```python
from build123d import *

# Parameters (mm, degrees)
BOSS_EXTRUDE1_DEPTH  = 15
BOSS_EXTRUDE8_DEPTH  = 10
SKETCH5_W            = 15
SKETCH5_H            = 15
BOSS_EXTRUDE10_DEPTH = 10
CUT_EXTRUDE4_DEPTH   = 10
BOSS_EXTRUDE11_DEPTH = 10


with BuildPart() as part:
    # Sketch1 → Boss-Extrude1 (new body)
    with BuildSketch(Plane.XY):
        Polygon((-20, -5), (-20, 5), (-10, 5), (-10, 10), (0, 10), (0, 0), (-10, 0), (-10, -5), align=None)
    extrude(amount=BOSS_EXTRUDE1_DEPTH)

    # Sketch2 → Boss-Extrude8 (add)
    with BuildSketch(Plane(origin=(-10, 0, 0), x_dir=(0, 0, -1), z_dir=(1, 0, 0))):
        Polygon((0, 0), (0, -5), (-15, 0), align=None)
    extrude(amount=BOSS_EXTRUDE8_DEPTH)

    # Sketch5 → Boss-Extrude10 (add)
    with BuildSketch(Plane(origin=(0, 0, 0), x_dir=(0, 0, -1), z_dir=(1, 0, 0))):
        with Locations((-7.5, 2.5)):
            Rectangle(SKETCH5_W, SKETCH5_H)
    extrude(amount=BOSS_EXTRUDE10_DEPTH)

    # Sketch6 → Cut-Extrude4 (cut)
    with BuildSketch(Plane(origin=(10, 0, 0), x_dir=(0, 0, -1), z_dir=(1, 0, 0))):
        Polygon((-15, -5), (0, 0), (0, -5), align=None)
    extrude(amount=-CUT_EXTRUDE4_DEPTH, mode=Mode.SUBTRACT)

    # Sketch7 → Boss-Extrude11 (add)
    with BuildSketch(Plane.ZY.offset(10)):
        Polygon((0, 5), (0, 15), (15, 5), align=None)
    extrude(amount=BOSS_EXTRUDE11_DEPTH)


solid = part.part
```
Model file for the job. Use its own axes, mm. A direction names the side the tool comes from. Give positions to 0.01 mm unless a question says otherwise; leave off trailing zeros. Write each loop counter-clockwise with the first axis right and the second up, starting at its lowest first coordinate (ties: lowest second). Pieces come first, ordered by that corner, then holes. Notation, with made-up numbers: (7, 33) -> (55, 33) arc R27 cw to (55, 58) -> close; hole circle Ø11 at (79, 16.25). An arc over 180 degrees is marked (long way). Use CSV: the item, a comma, the result in double quotes. Start each with the question number.
1) Two-plate mould, pull along X, no slides. Class faces 1 (the flat face through (-5.07, -2.535, 7.395)), 2 (the flat face through (0, 10, 8)), 3 (the flat face through (10, 4, 8)): released by +X, released by -X, zero draft, split by the parting line, or undercut.
2) Cut at B-B on z = 4.5. List the corners of the cut face in (x, y).
3) Cut at D-D on z = 11. List the corners of the cut face in (x, y).
4) Tool access for faces 4 (the flat face through (-10, 11, 2)), 5 (the flat face through (-14.93, 10.07, 7.395)), 6 (the flat face through (-10, -4, 11)): list every direction of +Z, -Z, +X, -X, +Y, -Y with a clear straight run to the whole face (end or side of a thin tool).
5) Drill centre lines: L1, parallel to X at y = -1.25, z = 13.5; L2, parallel to X at y = -2.5, z = 1; L3, parallel to X at y = 8, z = 11.75. Where is each one in solid material? Low to high.
6) Pin check, flat tips, straight feed: P1, Ø3, axis at x = 4.5, z = 13, coming from the -Y side; P2, Ø5.5, axis at y = 13.5, z = 4, coming from the +X side. Stop position of each tip, or through.
7) Cut at A-A on y = -3. List the corners of the cut face in (x, z), plus the area to 3 significant figures.
8) Cut at C-C on x = -9.5. List the corners of the cut face in (y, z), plus the area to 4 significant figures.
Final values:
1,face 1,"undercut"
1,face 2,"zero draft"
1,face 3,"released by +X"
2,outline,"(-20, -5) -> (-10, -5) -> (-10, -3.5) -> (0, -3.5) -> (0, -1.5) -> (10, -1.5) -> (10, 10) -> (-10, 10) -> (-10, 12) -> (-20, 12) -> close"
3,outline,"(-20, -5) -> (-10, -5) -> (-10, -1.33) -> (0, -1.33) -> (0, -3.67) -> (10, -3.67) -> (10, 10) -> (-10, 10) -> (-10, 7.67) -> (-20, 7.67) -> close"
4,face 4,"+Z, -Z, +X, +Y"
4,face 5,"+Z, -X, +Y"
4,face 6,"+Z, -Y"
5,L1,"x = -20 to -10, 0 to 10"
5,L2,"x = -20 to 0"
5,L3,"x = -10 to 10"
6,P1,"stops at y = -4.83"
6,P2,"stops at x = -10"
7,outline,"(-20, 0) -> (0, 0) -> (0, 6) -> (-10, 6) -> (-10, 15) -> (-20, 15) -> close; (0, 9) -> (10, 9) -> (10, 15) -> (0, 15) -> close"
7,area,"270 mm2"
8,outline,"(-5, 0) -> (10, 0) -> (10, 15) -> (0, 15) -> close"
8,area,"187.5 mm2"
